Geometry: final body of the model. Coordinates: model frame, mm. A direction names the side the tool comes from. Round coordinates to 2 decimals unless told otherwise and drop trailing zeros. Write each loop counter-clockwise with the first axis right and the second up, starting at its lowest first coordinate (ties: lowest second). Pieces come first, ordered by that corner, then holes. Notation, with made-up numbers: M -31.5,-11 L -22.5,-11 A10 ccw -22.5,8 Z; hole C 55,-28.5 d1. An arc over 180 degrees is marked long. Use one line per item in the form item = value. Start each with the question number.
Item 1: Section query D-D (y = -29). Return loops of the section in (x, z), and give its area (3 significant figures).
Item 2: Section query B-B (z = 48). Return loops of the section in (x, y) (3 decimals), and give its area (3 significant figures).
Item 3: Reachability of faces 1 (the flat face through (-28, 14.478, 145)), 2 (the flat face through (-28, -14.478, 145)), 3 (the cylindrical face through (-48.075, -51.934, 1.252)) from +Z, -Z, +X, -X, +Y, -Y: full face, straight path, thin tool, end or side. Return the list, or none.
Item 4: Section query A-A (y = 0). State how many separate pieces and enclosed holes the cut face has, and give its area (3 significant figures).
Item 5: Pull-direction query (X, two-part tool) for faces 4 (the flat face through (24.274, 0, 154)), 5 (the flat face through (31.386, 0, 154)), 6 (the flat face through (0, -32, 58.42)), 7 (the cylindrical face through (27.88, -1.209, 185.963)); classes: pulls with the +X half, pulls with the -X half, needs draft (parallel to the pull), parting line crosses it, or undercut.
Item 6: Pin query (flat end, axial travel): pin 1 Ø2 at (x, z) = (-26.5, 156.5) entering from -Y; pin 2 Ø23 at (y, z) = (1, 145.5) entering from +X; pin 3 Ø10 at (x, y) = (-15, -24.5) entering from +Z; pin 4 Ø15 at (y, z) = (0, 176.75) entering from -X. Return the tip coordinate at first contact, or that it passes through.
Item 7: Section query C-C (z = 159.5). Return loops of the section in (x, y), and give its area (3 significant figures).
Item 8: Ray query, probe 1 along Z at (x, y) = (-27.75, 0); probe 2 along X at (y, z) = (-41, 16); probe 3 along Y at (x, z) = (7.5, 21) (3 decimals). Return the intervals inside material, ascending.
from build123d import *

# Parameters (mm, degrees)
BOSS_EXTRUDE1_DEPTH     = 114.3
SKETCH2_W               = 55.88
SKETCH2_H               = 20.32
CUT_EXTRUDE1_DEPTH      = 58.42
SKETCH4_W               = 7.112
SKETCH4_H               = 28.956
BOSS_EXTRUDE2_DEPTH     = 83.82
CUT_EXTRUDE3_DEPTH      = 81.026
SKETCH8_R               = 9.290672209
CUT_EXTRUDE4_DEPTH      = 81.026
FILLET1_R               = 2.54
CUT_EXTRUDE_THIN1_DEPTH = 2.54


with BuildPart() as part:
    # Sketch1 → Boss-Extrude1 (new body)
    with BuildSketch(Plane.XY):
        with BuildLine():
            Line((45.101951145, 57.785), (-45.101951145, 57.785))
            ThreePointArc((-45.101951145, 57.785), (-51.38813043, 55.181179285), (-53.991951145, 48.895))
            Line((-53.991951145, 48.895), (-53.991951145, -48.895))
            ThreePointArc((-53.991951145, -48.895), (-51.38813043, -55.181179285), (-45.101951145, -57.785))
            Line((-45.101951145, -57.785), (45.101951145, -57.785))
            ThreePointArc((45.101951145, -57.785), (51.38813043, -55.181179285), (53.991951145, -48.895))
            Line((53.991951145, -48.895), (53.991951145, 48.895))
            ThreePointArc((53.991951145, 48.895), (51.38813043, 55.181179285), (45.101951145, 57.785))
        make_face()
    extrude(amount=BOSS_EXTRUDE1_DEPTH)

    # Sketch2 → Cut-Extrude1 (cut)
    with BuildSketch(Plane(origin=(0, 0, 0), x_dir=(-1, 0, 0), z_dir=(0, 0, -1))):
        with Locations((0, -32.385)):
            Rectangle(SKETCH2_W, SKETCH2_H)
    extrude(amount=-CUT_EXTRUDE1_DEPTH, mode=Mode.SUBTRACT)

    # Sketch4 → Boss-Extrude2 (add)
    with BuildSketch(Plane.XY.offset(114.3)):
        with Locations((-27.829951145, 0)):
            Rectangle(SKETCH4_W, SKETCH4_H)
        with Locations((27.829951145, 0)):
            Rectangle(SKETCH4_W, SKETCH4_H)
    extrude(amount=BOSS_EXTRUDE2_DEPTH)

    # Sketch7 → Cut-Extrude3 (cut)
    with BuildSketch(Plane(origin=(31.385951145, 0, 0), x_dir=(0, 0, -1), z_dir=(1, 0, 0))):
        Polygon((-214.942074504, -34.200153794), (-240.17713944, 1.162141148), (-200.137312033, 42.544769544), (-200.137312033, 40.508920027), (-166.132146275, 16.934056733), (-214.942074504, 5.644685578), (-204.648824334, -5.976725906), (-166.132146275, -17.930177717), align=None)
    extrude(amount=-CUT_EXTRUDE3_DEPTH, mode=Mode.SUBTRACT)

    # Sketch8 → Cut-Extrude4 (cut)
    with BuildSketch(Plane(origin=(31.385951145, 0, 0), x_dir=(0, 0, -1), z_dir=(1, 0, 0))):
        with Locations(Location((-176.750979796, 0, 0), (0, 0, 90))):
            Circle(SKETCH8_R)
    extrude(amount=-CUT_EXTRUDE4_DEPTH, mode=Mode.SUBTRACT)

    # Fillet1
    fillet1_edges = [part.edges().sort_by_distance(p)[0] for p in [
        (31.385951145, 0.766296382, 198.12),
        (24.273951145, 0.766296382, 198.12),
        (-31.385951145, 0.766296382, 198.12),
        (-24.273951145, 0.766296382, 198.12),
    ]]
    fillet(fillet1_edges, radius=FILLET1_R)

    # Sketch9 → Cut-Extrude-Thin1 (cut)
    with BuildSketch(Plane(origin=(0, 0, 0), x_dir=(-1, 0, 0), z_dir=(0, 0, -1))):
        with BuildLine():
            Line((-45.101951145, -53.146398513), (45.101951145, -53.146398513))
            ThreePointArc((45.101951145, -53.146398513), (48.108143863, -51.901192718), (49.353349658, -48.895))
            Line((49.353349658, -48.895), (49.353349658, 48.895))
            ThreePointArc((49.353349658, 48.895), (48.108143863, 51.901192718), (45.101951145, 53.146398513))
            Line((45.101951145, 53.146398513), (-45.101951145, 53.146398513))
            ThreePointArc((-45.101951145, 53.146398513), (-48.108143863, 51.901192718), (-49.353349658, 48.895))
            Line((-49.353349658, 48.895), (-49.353349658, -48.895))
            ThreePointArc((-49.353349658, -48.895), (-48.108143863, -51.901192718), (-45.101951145, -53.146398513))
        make_face()
        with BuildLine():
            Line((-45.101951145, -52.638398513), (45.101951145, -52.638398513))
            ThreePointArc((45.101951145, -52.638398513), (47.748933618, -51.541982473), (48.845349658, -48.895))
            Line((48.845349658, -48.895), (48.845349658, 48.895))
            ThreePointArc((48.845349658, 48.895), (47.748933618, 51.541982473), (45.101951145, 52.638398513))
            Line((45.101951145, 52.638398513), (-45.101951145, 52.638398513))
            ThreePointArc((-45.101951145, 52.638398513), (-47.748933618, 51.541982473), (-48.845349658, 48.895))
            Line((-48.845349658, 48.895), (-48.845349658, -48.895))
            ThreePointArc((-48.845349658, -48.895), (-47.748933618, -51.541982473), (-45.101951145, -52.638398513))
        make_face(mode=Mode.SUBTRACT)
    extrude(amount=-CUT_EXTRUDE_THIN1_DEPTH, mode=Mode.SUBTRACT)


solid = part.part
Working result:
q1.outline = M -53.99,0 L -49.35,0 L -49.35,2.54 L -48.85,2.54 L -48.85,0 L -27.94,0 L -27.94,58.42 L 27.94,58.42 L 27.94,0 L 48.85,0 L 48.85,2.54 L 49.35,2.54 L 49.35,0 L 53.99,0 L 53.99,114.3 L -53.99,114.3 Z
q1.area = 9,080 mm²
q2.outline = M -53.992,-48.895 A8.89 ccw -45.102,-57.785 L 45.102,-57.785 A8.89 ccw 53.992,-48.895 L 53.992,48.895 A8.89 ccw 45.102,57.785 L -45.102,57.785 A8.89 ccw -53.992,48.895 Z; hole M -27.94,-42.545 L 27.94,-42.545 L 27.94,-22.225 L -27.94,-22.225 Z
q2.area = 11,300 mm²
q3.face_1 = +Z, +X, -X, +Y
q3.face_2 = +Z, +X, -X, -Y
q3.face_3 = -Z
q4.separate_pieces = 3
q4.enclosed_holes = 0
q4.area = 13,300 mm²
q5.face_4 = undercut
q5.face_5 = pulls with the +X half
q5.face_6 = undercut
q5.face_7 = needs draft
q6.pin_1 = -14.48
q6.pin_2 = 31.39
q6.pin_3 = 114.3
q6.pin_4 = through
q7.outline = M -31.39,-14.48 L -24.27,-14.48 L -24.27,14.48 L -31.39,14.48 Z; M 24.27,-14.48 L 31.39,-14.48 L 31.39,14.48 L 24.27,14.48 Z
q7.area = 412 mm²
q8.probe_1 = 0 to 167.46, 186.04 to 198.12
q8.probe_2 = -53.99 to -27.94, 27.94 to 53.99
q8.probe_3 = -57.785 to -42.545, -22.225 to 57.785
